Part model, mm, in its own coordinate system. A direction names the side the tool comes from. Round coordinates to 2 decimals unless told otherwise and drop trailing zeros. Write each loop counter-clockwise with the first axis right and the second up, starting at its lowest first coordinate (ties: lowest second). Pieces come first, ordered by that corner, then holes.
1) Pull direction X, two halves, no side cores. Call faces 1 (the flat face through (-21, -183.75, 0)), 2 (the flat face through (-110, -258, 0)), 3 (the cylindrical face through (-7.129, -259.982, -0.28)), 4 (the cylindrical face through (-60, -255, 0)): +X half, -X half, draft (parallel to the pull), parting line (faces both ways), or undercut.
2) Which spindle directions (+Z, -Z, +X, -X, +Y, -Y) get a long thin tool onto all of the face, cutting with end or side? Do faces 5 (the flat face through (-70, -116, 0)), 6 (the cylindrical face through (-102.119, -12.325, -1.915)), 7 (the flat face through (-25, -155, 0)), 8 (the flat face through (-110, -110, 0)), 9 (the flat face through (-42, -255, -12.5)). Say none if no direction does.
3) Saw through at B-B on x = -140. Write the cut outline in (y, z), and give its area (3 significant figures).
4) Saw through at A-A on x = -97.5. Write the cut outline in (y, z) (3 decimals), and give its area (3 significant figures).
5) Saw through at C-C on y = -40. Write the cut outline in (x, z), and give its area (3 significant figures).
6) Drill centre lines: L1, parallel to Y at x = -63, z = -17; L2, parallel to Y at x = -81, z = 0 (3 decimals); L3, parallel to Z at x = -182.5, y = -13.75. Where is each one in solid material? Low to high.
7) Flat gauge pins, fed straight in: pin 1 (9 mm diameter, centred on x = -19.5, z = -3.5, fed in from +Y); pin 2 (2.5 mm diameter, centred on x = -20.5, z = -8, fed in from -Y); pin 3 (2 mm diameter, centred on y = -234, z = -0.5, fed in from -X); pin 4 (24 mm diameter, centred on x = -140, z = 0, fed in from -Y). Where does each tip first touch, or does it go through?
8) Saw through at D-D on x = -166.5. Write the cut outline in (y, z), and give its area (3 significant figures).
```python
from build123d import *

# Parameters (mm, degrees)
BOSS_EXTRUDE1_DEPTH = 20
BOSS_EXTRUDE2_DEPTH = 25
SKETCH3_R           = 15
SKETCH3_R_2         = 5
CUT_EXTRUDE1_DEPTH  = 25
FILLET1_R           = 25
SKETCH4_R           = 6
CUT_EXTRUDE2_DEPTH  = 40
SKETCH5_W           = 40
SKETCH5_H           = 16.5
CUT_EXTRUDE3_DEPTH  = 8
RIB1_REACH          = 339.611
SKETCH6_WALL_W      = 733.123885092
SKETCH6_WALL_H      = 25
CUT_EXTRUDE4_DEPTH  = 25
SKETCH8_W           = 9
SKETCH8_H           = 24
CUT_EXTRUDE5_DEPTH  = 8


with BuildPart() as part:
    # Sketch1 → Boss-Extrude1 (new, symmetric)
    with BuildSketch(Plane.XY):
        Polygon((-185, 0), (0, 0), (0, -267.5), (-110, -267.5), (-110, -242.5), (-25, -242.5), (-25, -125), (-110, -125), (-110, -100), (-25, -100), (-25, -25), (-185, -25), align=None)
    extrude(amount=BOSS_EXTRUDE1_DEPTH, both=True)

    # Sketch2 → Boss-Extrude2 (add)
    with BuildSketch(Plane(origin=(0, 0, 0), x_dir=(1, 0, 0), z_dir=(0, 1, 0))):
        with BuildLine():
            Line((-185, 20), (-185, -20))
            ThreePointArc((-185, -20), (-205, 0), (-185, 20))
        make_face()
    extrude(amount=-BOSS_EXTRUDE2_DEPTH)

    # Sketch3 → Cut-Extrude1 (cut)
    with BuildSketch(Plane(origin=(0, 0, 0), x_dir=(1, 0, 0), z_dir=(0, 1, 0))):
        with Locations(Location((-140, 0, 0), (0, 0, 180))):
            Circle(SKETCH3_R)
        with Locations(Location((-182.5, 0, 0), (0, 0, 180))):
            Circle(SKETCH3_R_2)
        with Locations(Location((-97.5, 0, 0), (0, 0, 180))):
            Circle(SKETCH3_R_2)
    extrude(amount=-CUT_EXTRUDE1_DEPTH, mode=Mode.SUBTRACT)

    # Fillet1
    fillet1_edges = [part.edges().sort_by_distance(p)[0] for p in [
        (0, 0, 0),
        (0, -267.5, 0),
    ]]
    fillet(fillet1_edges, radius=FILLET1_R)

    # Sketch4 → Cut-Extrude2 (cut)
    with BuildSketch(Plane.ZY.offset(110)):
        with Locations((0, -251.225)):
            Circle(SKETCH4_R)
        with Locations(Location((0, -116.275, 0), (0, 0, 180))):
            Circle(SKETCH4_R)
    extrude(amount=-CUT_EXTRUDE2_DEPTH, mode=Mode.SUBTRACT)

    # Sketch5 → Cut-Extrude3 (cut)
    with BuildSketch(Plane.ZY.offset(25)):
        with Locations((0, -70.75)):
            Rectangle(SKETCH5_W, SKETCH5_H)
        with Locations((0, -192)):
            Rectangle(SKETCH5_W, SKETCH5_H)
    extrude(amount=-CUT_EXTRUDE3_DEPTH, mode=Mode.SUBTRACT)

    # Sketch6 wall → Rib1 (add, up to next)
    with BuildSketch(Plane(origin=(-50, -37.5, 0), x_dir=(0.894427191, -0.4472135955, 0), z_dir=(0.4472135955, 0.894427191, 0)), mode=Mode.PRIVATE) as rib1_sk1:
        Rectangle(SKETCH6_WALL_W, SKETCH6_WALL_H)
    rib1_tool1 = extrude(rib1_sk1.sketch, amount=RIB1_REACH, mode=Mode.PRIVATE) - part.part
    add(rib1_tool1.solids().sort_by_distance((-50, -37.5, 0))[0])

    # Sketch7 → Cut-Extrude4 (cut)
    with BuildSketch(Plane.XZ.offset(267.5)):
        with BuildLine():
            Line((-47.5, 12.5), (-37.5, 12.5))
            ThreePointArc((-37.5, 12.5), (-25, 0), (-37.5, -12.5))
            Line((-37.5, -12.5), (-47.5, -12.5))
            ThreePointArc((-47.5, -12.5), (-60, 0), (-47.5, 12.5))
        make_face()
    extrude(amount=-CUT_EXTRUDE4_DEPTH, mode=Mode.SUBTRACT)

    # Sketch8 → Cut-Extrude5 (cut)
    with BuildSketch(Plane.XZ.offset(125)):
        with Locations((-42.5, 0)):
            Rectangle(SKETCH8_W, SKETCH8_H)
    extrude(amount=-CUT_EXTRUDE5_DEPTH, mode=Mode.SUBTRACT)


solid = part.part
```
Completed:
1. face 1: draft
1. face 2: -X half
1. face 3: +X half
1. face 4: undercut
2. face 5: -X
2. face 6: +Y
2. face 7: +Z, -Z, -X
2. face 8: +Z, -Z, -X, -Y
2. face 9: -Y
3. outline: (-25, -20) - (0, -20) - (0, -15) - (-25, -15) - close; (-25, 15) - (0, 15) - (0, 20) - (-25, 20) - close
3. area: 250 mm2
4. outline: (-267.5, -20) - (-242.5, -20) - (-242.5, 20) - (-267.5, 20) - close; (-125, -20) - (-100, -20) - (-100, 20) - (-125, 20) - close; (-25, -20) - (0, -20) - (0, -5) - (-25, -5) - close; (-25, 5) - (0, 5) - (0, 20) - (-25, 20) - close; hole circle Ø12 at (-251.225, 0); hole circle Ø12 at (-116.275, 0)
4. area: 2,520 mm2
5. outline: (-45, -12.5) - (-25, -12.5) - (-25, -20) - (0, -20) - (0, 20) - (-25, 20) - (-25, 12.5) - (-45, 12.5) - close
5. area: 1,500 mm2
6. L1: y = -267.5 to -242.5, -125 to -100, -25 to 0
6. L2: y = -267.5 to -257.225, -245.225 to -242.5, -125 to -122.275, -110.275 to -100, -25 to 0
6. L3: z = -20 to -5, 5 to 20
7. pin 1: stops at y = -0.02
7. pin 2: stops at y = -267.29
7. pin 3: stops at x = -25
7. pin 4: passes through
8. outline: (-25, -20) - (0, -20) - (0, 20) - (-25, 20) - close
8. area: 1,000 mm2
